from build123d import *

# Parameters (mm, degrees)
SKETCH1_W           = 19.05
SKETCH1_H           = 19.05
SKETCH1_W_2         = 15.875
SKETCH1_H_2         = 15.875
BOSS_EXTRUDE1_DEPTH = 914.4
SKETCH2_R           = 2.75
CUT_EXTRUDE1_DEPTH  = 20.05
CUT_EXTRUDE2_REACH  = 21.05
SKETCH3_R           = 4.255
SKETCH4_OUTSIDE_W   = 204.01
SKETCH4_OUTSIDE_H   = 1099.36
SKETCH4_OUTSIDE_W_2 = 19.05
SKETCH4_OUTSIDE_H_2 = 203.2
CUT_EXTRUDE3_DEPTH  = 20.05
SKETCH5_R           = 2.75
CUT_EXTRUDE4_DEPTH  = 20.05


with BuildPart() as part:
    # Sketch1 → Boss-Extrude1 (new body)
    with BuildSketch(Plane(origin=(0, 0, 0), x_dir=(1, 0, 0), z_dir=(0, 1, 0))):
        with Locations((9.525, 9.525)):
            Rectangle(SKETCH1_W, SKETCH1_H)
        with Locations((9.525, 9.525)):
            Rectangle(SKETCH1_W_2, SKETCH1_H_2, mode=Mode.SUBTRACT)
    extrude(amount=BOSS_EXTRUDE1_DEPTH)

    # Sketch2 → Cut-Extrude1 (cut, through all)
    with BuildSketch(Plane.XY):
        with Locations((9.525, 906.4)):
            Circle(SKETCH2_R)
        with Locations((9.525, 891.4)):
            Circle(SKETCH2_R)
    extrude(amount=-CUT_EXTRUDE1_DEPTH, mode=Mode.SUBTRACT)

    # Sketch3 → Cut-Extrude2 (cut, up to next)
    with BuildSketch(Plane(origin=(0, 0, -19.05), x_dir=(-1, 0, 0), z_dir=(0, 0, -1)), mode=Mode.PRIVATE) as cut_extrude2_sk1:
        with Locations((-9.525, 906.4)):
            Circle(SKETCH3_R)
    cut_extrude2_tool1 = extrude(cut_extrude2_sk1.sketch, amount=-CUT_EXTRUDE2_REACH, mode=Mode.PRIVATE) & part.part
    add(cut_extrude2_tool1.solids().sort_by_distance((9.525, 906.4, -19.05))[0], mode=Mode.SUBTRACT)
    # Sketch3 → Cut-Extrude2 (cut, up to next)
    with BuildSketch(Plane(origin=(0, 0, -19.05), x_dir=(-1, 0, 0), z_dir=(0, 0, -1)), mode=Mode.PRIVATE) as cut_extrude2_sk2:
        with Locations((-9.525, 891.4)):
            Circle(SKETCH3_R)
    cut_extrude2_tool2 = extrude(cut_extrude2_sk2.sketch, amount=-CUT_EXTRUDE2_REACH, mode=Mode.PRIVATE) & part.part
    add(cut_extrude2_tool2.solids().sort_by_distance((9.525, 891.4, -19.05))[0], mode=Mode.SUBTRACT)

    # Sketch4 outside → Cut-Extrude3 (cut, through all)
    with BuildSketch(Plane.XY):
        with Locations((9.525, 457.2)):
            Rectangle(SKETCH4_OUTSIDE_W, SKETCH4_OUTSIDE_H)
        with Locations((9.525, 660.4)):
            Rectangle(SKETCH4_OUTSIDE_W_2, SKETCH4_OUTSIDE_H_2, mode=Mode.SUBTRACT)
    extrude(amount=-CUT_EXTRUDE3_DEPTH, mode=Mode.SUBTRACT)

    # Sketch5 → Cut-Extrude4 (cut, through all)
    with BuildSketch(Plane.XY):
        with Locations((9.52, 735.8)):
            Circle(SKETCH5_R)
        with Locations((9.52, 705.8)):
            Circle(SKETCH5_R)
        with Locations((9.52, 585)):
            Circle(SKETCH5_R)
        with Locations((9.52, 615)):
            Circle(SKETCH5_R)
    extrude(amount=-CUT_EXTRUDE4_DEPTH, mode=Mode.SUBTRACT)


solid = part.part
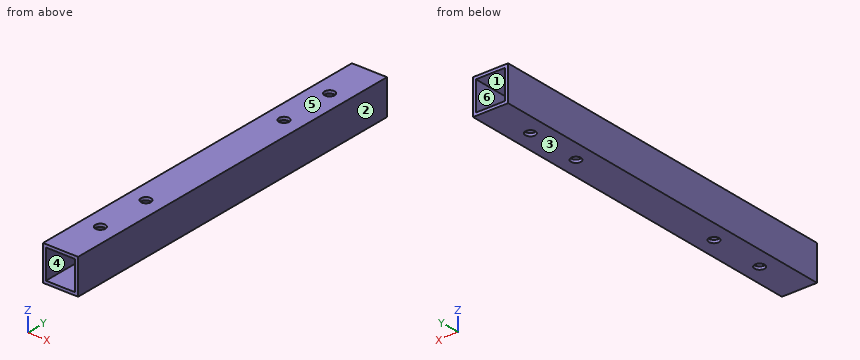
Can you work these out from the model? Positions are in its coordinate system, mm. Face numbers are marked on the shaded views. A direction names the side the tool comes from. Give positions to 0.01 mm unless a question says otherwise; leave off trailing zeros. Order: outer loops, then holes, each group sorted by start corner. A loop starts at its lowest first (then second) coordinate and runs counter-clockwise, first axis right, second up. Notation, with made-up numbers: M -12,74.5 L 27,74.5 A23 ccw 27,106.5 Z; hole C 42.25,17.5 d9. An arc over 180 degrees is marked long. One line per item, written item: value.
Item 1: If we section it at A-A on y = 715: Write out the boundary of the cut face in (x, z).
Verdict:
outline: M 0,-19.05 L 19.05,-19.05 L 19.05,0 L 0,0 Z; hole M 1.59,-17.46 L 17.46,-17.46 L 17.46,-1.59 L 1.59,-1.59 Z
Item 2: For the marked faces 1 and 2, which set-ups out of +Z, -Z, +X, -X, +Y, -Y let a thin tool reach every point of the face, with its end or its side?
Verdict:
face 1: +Y, -Y
face 2: +Z, -Z, +X, +Y, -Y
Item 3: If we section it at C-C on x = 15: Write out the boundary of the cut face in (y, z), and give its area (3 significant figures).
Verdict:
outline: M 558.8,-19.05 L 762,-19.05 L 762,-17.46 L 558.8,-17.46 Z; M 558.8,-1.59 L 762,-1.59 L 762,0 L 558.8,0 Z
area: 645 mm2
Item 4: Please list where these lines run through material, in increasing order: line 1 (Y direction, x = 9.52, z = -0.9); line 2 (X direction, y = 687, z = -9.75); line 3 (X direction, y = 615, z = -1).
Verdict:
line 1: 558.8 to 582.25, 587.75 to 612.25, 617.75 to 703.05, 708.55 to 733.05, 738.55 to 762
line 2: 0 to 1.59, 17.46 to 19.05
line 3: 0 to 6.77, 12.27 to 19.05
Item 5: For pin 1 (2 mm diameter, centred on y = 668, z = -3.5, fed in from -X); pin 2 (1 mm diameter, centred on x = 8, y = 706.5, fed in from +Z), each with a flat end and sliding along its axis, tell me the tip position at first contact or that it passes through.
Verdict:
pin 1: x = 0
pin 2: through
Item 6: If we section it at B-B on z = -9.5: Write out the boundary of the cut face in (x, y), and give its area (3 significant figures).
Verdict:
outline: M 0,558.8 L 1.59,558.8 L 1.59,762 L 0,762 Z; M 17.46,558.8 L 19.05,558.8 L 19.05,762 L 17.46,762 Z
area: 645 mm2
Item 7: If we mould it in two halves opening along Z, with no side actions, what happens to the marked faces 3, 4, 5 and 6? For each: pulls with the +Z half, pulls with the -Z half, needs draft (parallel to the pull), parting line crosses it, or undercut.
Verdict:
face 3: pulls with the -Z half
face 4: undercut
face 5: pulls with the +Z half
face 6: undercut
